```python
from build123d import *

# Parameters (mm, degrees)
SKETCH_1_R                   = 59
SKETCH_1_R_2                 = 53
EXTRUDE_1_DEPTH              = 3.975
SKETCH_2_R                   = 59
SKETCH_2_R_2                 = 50.5
EXTRUDE_2_DEPTH              = 2
HOLE_WIZARD_M3_1_D           = 2.5
HOLE_WIZARD_M3_1_CSINK_D     = 3.05
HOLE_WIZARD_M3_1_CSINK_ANGLE = 90
PATTERN_CIRCULAR_1_COUNT     = 8


with BuildPart() as part:
    # 草图1 → 凸台-拉伸1 (new, symmetric)
    with BuildSketch(Plane.XY):
        Circle(SKETCH_1_R)
        Circle(SKETCH_1_R_2, mode=Mode.SUBTRACT)
    extrude(amount=EXTRUDE_1_DEPTH, both=True)

    # 草图2 → 凸台-拉伸2 (add)
    with BuildSketch(Plane(origin=(0, 0, -3.975), x_dir=(-1, 0, 0), z_dir=(0, 0, -1))):
        Circle(SKETCH_2_R)
        Circle(SKETCH_2_R_2, mode=Mode.SUBTRACT)
    extrude(amount=EXTRUDE_2_DEPTH)

    # M3 螺纹孔1 (through all)
    with Locations(Plane.XY.offset(3.975)):
        with Locations((0, 56)):
            hole_wizard_m3_1 = CounterSinkHole(HOLE_WIZARD_M3_1_D / 2, HOLE_WIZARD_M3_1_CSINK_D / 2, counter_sink_angle=HOLE_WIZARD_M3_1_CSINK_ANGLE)

    # 阵列(圆周)1: M3 螺纹孔1 ×8 about axis
    pattern_circular_1_axis = Axis((0, 0, 0), (0, 0, 1))
    for i in range(1, PATTERN_CIRCULAR_1_COUNT):
        add(hole_wizard_m3_1.rotate(pattern_circular_1_axis, i * 360 / PATTERN_CIRCULAR_1_COUNT), mode=Mode.SUBTRACT)


solid = part.part
```
Part model, mm, in its own coordinate system. A direction names the side the tool comes from. Round coordinates to 2 decimals unless told otherwise and drop trailing zeros. Write each loop counter-clockwise with the first axis right and the second up, starting at its lowest first coordinate (ties: lowest second). Pieces come first, ordered by that corner, then holes.
Item 1: Two-plate mould, pull along X, no slides. Class faces 1 (the cylindrical face through (28, 45, 0)), 2 (the flat face through (-48.35, 22.13, 3.975)): +X half, -X half, draft (parallel to the pull), parting line (faces both ways), or undercut.
Results:
face 1: undercut
face 2: draft
Item 2: Cut at B-B, the plane x = 3. Give the cut face in (y, z) (3 decimals).
Results:
outline: (-58.924, -5.975) - (-50.411, -5.975) - (-50.411, -3.975) - (-52.915, -3.975) - (-52.915, 3.975) - (-58.924, 3.975) - close; (50.411, -5.975) - (58.924, -5.975) - (58.924, 3.975) - (52.915, 3.975) - (52.915, -3.975) - (50.411, -3.975) - close
Item 3: Drop flat-ended pins along their axis: pin 1 Ø5 at (x, z) = (25.5, -1.5) entering from +Y; pin 2 Ø5 at (y, z) = (38.5, -1.5) entering from +X; pin 3 Ø3 at (x, y) = (39.6, -39.6) entering from -Z (3 decimals); pin 4 Ø3 at (x, y) = (0, 56) entering from +Z. Give the stop position or say it passes through.
Results:
pin 1: stops at y = 54.33
pin 2: stops at x = 46.74
pin 3: stops at z = -5.975
pin 4: stops at z = 3.95
Item 4: Cut at A-A, the plane y = -29. Give the cut face in (x, z) (3 decimals).
Results:
outline: (-51.381, -5.975) - (-41.343, -5.975) - (-41.343, -3.975) - (-44.362, -3.975) - (-44.362, 3.975) - (-51.381, 3.975) - close; (41.343, -5.975) - (51.381, -5.975) - (51.381, 3.975) - (44.362, 3.975) - (44.362, -3.975) - (41.343, -3.975) - close
Item 5: Probe L1, parallel to Y at x = 0, z = -1; L2, parallel to Y at x = -39.5, z = -1.25; L3, parallel to Y at x = -24, z = 1.25. List the from-to ranges inside material, lowest first.
Results:
L1: y = -59 to -57.25, -54.75 to -53, 53 to 54.75, 57.25 to 59
L2: y = -43.83 to -40.84, -38.35 to -35.34, 35.34 to 38.35, 40.84 to 43.83
L3: y = -53.9 to -47.25, 47.25 to 53.9
Item 6: Which spindle directions (+Z, -Z, +X, -X, +Y, -Y) get a long thin tool onto all of the face, cutting with end or side? Do faces 3 (the flat face through (-47, -19, -3.975)), 4 (the flat face through (18, -48, -5.975)). Say none if no direction does.
Results:
face 3: +Z
face 4: -Z, +X, -X, +Y, -Y
Item 7: Cut at C-C, the plane z = 0.75. Count the separate pieces of the cut face and the enclosed holes in it, plus the area to 3 significant figures.
Results:
separate pieces: 1
enclosed holes: 9
area: 2,070 mm2
